Can you work these out from the model? Positions are in its coordinate system, mm. A direction names the side the tool comes from. Round coordinates to 2 decimals unless told otherwise and drop trailing zeros. Loops run counter-clockwise (first coordinate to the right, second up) from the corner with the lowest first, then second, coordinate; pieces in that order, holes last.
(1) I want a section at A-A on z = 64.5. Write out the boundary of the cut face in (x, y).
(2) Will these pins go through, and if not, where does the flat tip stop? pin 1 Ø4 at (y, z) = (4, 5.5) entering from -X; pin 2 Ø1.5 at (y, z) = (3, 7) entering from +X.
(3) I want a section at C-C on y = 3.25. Write out the boundary of the cut face in (x, z), plus the area to 3 significant figures.
(4) Which directions (+Z, -Z, +X, -X, +Y, -Y) give clear straight access to the entire face, cutting with the end or side of a thin tool? Please do faces 1 (the face through (-1.25, 3, 5)), 2 (the face through (1.25, 3, 5)).
(5) If I drill on line 1 along Z through (x, y) = (-0.7, 5.5); line 2 along Y through (x, z) = (-0.05, 52); line 3 along Y through (x, z) = (0.85, 197.5), over which ranges is the centre line in solid material (lowest first)?
(6) I want a section at B-B on x = 0. Write out the boundary of the cut face in (y, z).
from build123d import *

# Parameters (mm, degrees)
SKETCH1_R           = 1.5
BOSS_EXTRUDE1_DEPTH = 212.4
BOSS_EXTRUDE2_DEPTH = 10


with BuildPart() as part:
    # Sketch1 → Boss-Extrude1 (new body)
    with BuildSketch(Plane.XY):
        Circle(SKETCH1_R)
    extrude(amount=BOSS_EXTRUDE1_DEPTH)

    # Sketch2 → Boss-Extrude2 (add)
    with BuildSketch(Plane(origin=(0, 0, 0), x_dir=(-1, 0, 0), z_dir=(0, 0, -1))):
        with BuildLine():
            Line((-1.25, 5.829156198), (-1.25, 0.829156198))
            ThreePointArc((-1.25, 0.829156198), (0, 1.5), (1.25, 0.829156198))
            Line((1.25, 0.829156198), (1.25, 5.829156198))
            Line((1.25, 5.829156198), (-1.25, 5.829156198))
        make_face()
    extrude(amount=-BOSS_EXTRUDE2_DEPTH)


solid = part.part
Filled sheet:
1. outline: circle Ø3 at (0, 0)
2. pin 1: stops at x = -1.25
2. pin 2: stops at x = 1.25
3. outline: (-1.25, 0) - (1.25, 0) - (1.25, 10) - (-1.25, 10) - close
3. area: 25.0 mm2
4. face 1: +Z, -Z, -X, +Y
4. face 2: +Z, -Z, +X, +Y
5. line 1: z = 0 to 10
5. line 2: y = -1.5 to 1.5
5. line 3: y = -1.24 to 1.24
6. outline: (-1.5, 0) - (5.83, 0) - (5.83, 10) - (1.5, 10) - (1.5, 212.4) - (-1.5, 212.4) - close
